The listing builds one solid part. Answer for the finished solid, in the listing's coordinates (mm). Face numbers are marked on the shaded views. A direction names the side the tool comes from. Round coordinates to 2 decimals unless told otherwise and drop trailing zeros. Order: outer loops, then holes, each group sorted by start corner. A loop starts at its lowest first (then second) coordinate and runs counter-clockwise, first axis right, second up. Notation, with made-up numbers: (66.5, -27.75) - (92.5, -27.75) arc R10 cw to (92.5, -15.75) - close; hole circle Ø4 at (75.5, 38). An arc over 180 degrees is marked (long way). One line per item, written item: value. Start each with the question number.
1. A tool of negligible diameter and unlimited length cuts with its end or side. For the marked faces 1, 2 and 3, from which of +Z, -Z, +X, -X, +Y, -Y can it reach the whole face along a straight path? Write none if from no direction.
2. Section C-C, the plane x = 12 is taken. Give the vertices of the cut face in (y, z), then the cut area to 3 significant figures.
3. Section A-A, the plane y = 0 is taken. Give the vertices of the cut face in (x, z), then the cut area to 3 significant figures.
4. Section D-D, the plane z = -6 is taken. Give the vertices of the cut face in (x, y).
5. Straight lines are drawn through the part: line 1 (X direction, y = 0, z = 5.25); line 2 (X direction, y = 0, z = 9.95); line 3 (Y direction, x = 0.5, z = 5.5). For each, find the intervals that lie inside material, in ascending order.
6. Flat-ended cylindrical pins translate along their axes: P1, Ø2, axis at x = 11, y = 11.5, coming from the -Z side; P2, Ø1.5, axis at x = -8.5, z = -16.5, coming from the -Y side; P3, Ø9, axis at x = 3, y = -2, coming from the +Z side. Find the tip coordinate at first contact, or state that the pin passes through.
7. For a pull along X with two mould halves and no side action, classify the marked faces 4, 5 and 6 as released by +X, released by -X, zero draft, split by the parting line, or undercut.
Autodesk Inventor part; units mm, degrees
ref_plane "YZ Plane" through (0, 0, 0) normal (1, 0, 0) x (0, 1, 0)
ref_plane "XZ Plane" through (0, 0, 0) normal (0, 1, 0) x (-1, 0, 0)
ref_plane "XY Plane" through (0, 0, 0) normal (0, 0, 1) x (1, 0, 0)
sketch "Sketch5" plane through (0, 0, 0) normal (1, 0, 0) x (0, 1, 0)
  line L0 (0, 0) -> (17.5, 0)
  line L1 (17.5, 0) -> (17.5, 12.8)
  line L2 (17.5, 12.8) -> (14, 12.8)
  line L3 (14, 12.8) -> (14, 10.3)
  line L4 (14, 10.3) -> (14.7, 10.3)
  line L5 (14.7, 10.3) -> (14.7, 9)
  line L6 (14.7, 9) -> (14, 9)
  line L7 (14, 9) -> (14, 2)
  line L8 (14, 2) -> (8, 2)
  line L9 (8, 2) -> (8, 0)
  line L10 (0, 0) -> (0, 12.8)
  line L11 (9.5, 0) -> (9.5, -25)
  line L12 (9.5, -25) -> (0, -25)
  line L13 (0, -25) -> (0, 0)
  line L14 (8, -25) -> (8, 0)
  dimension "d19" = 17.5
  dimension "d20" = 2.5
  dimension "d21" = 1.3
  dimension "d22" = 7
  dimension "d23" = 2
  dimension "d24" = 14.7
  dimension "d25" = 14
  dimension "d26" = 8
  dimension "d28" = 25
  dimension "d29" = 9.5
  dimension "d30" = 8
revolve "Revolution1" add sketch "Sketch5" angle 360 about axis through (0, 0, 0) along (0, 0, 1) contours L9 L8 L7 L6 L5 L4 L3 L2 L1 L0 | L0 L11 L12 L14
properties part number "P502" material "Aluminum 6061"
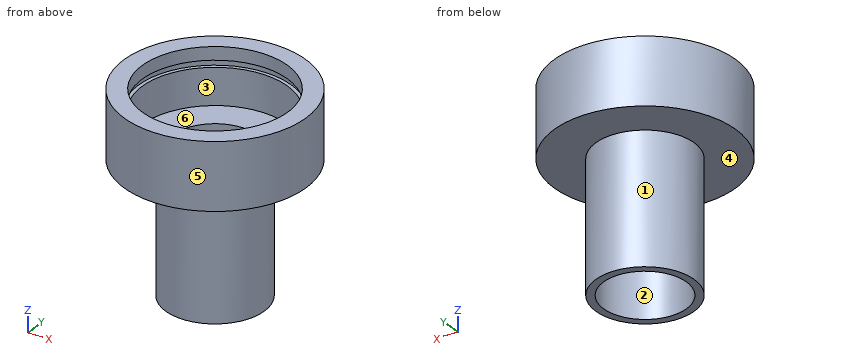
Answer list:
1. face 1: -Z
1. face 2: +Z, -Z
1. face 3: +Z
2. outline: (-12.74, 0) - (12.74, 0) - (12.74, 12.8) - (7.21, 12.8) - (7.21, 10.3) - (8.49, 10.3) - (8.49, 9) - (7.21, 9) - (7.21, 2) - (-7.21, 2) - (-7.21, 9) - (-8.49, 9) - (-8.49, 10.3) - (-7.21, 10.3) - (-7.21, 12.8) - (-12.74, 12.8) - close
2. area: 167 mm²
3. outline: (-17.5, 0) - (-9.5, 0) - (-9.5, -25) - (-8, -25) - (-8, 2) - (-14, 2) - (-14, 9) - (-14.7, 9) - (-14.7, 10.3) - (-14, 10.3) - (-14, 12.8) - (-17.5, 12.8) - close; (8, -25) - (9.5, -25) - (9.5, 0) - (17.5, 0) - (17.5, 12.8) - (14, 12.8) - (14, 10.3) - (14.7, 10.3) - (14.7, 9) - (14, 9) - (14, 2) - (8, 2) - close
3. area: 187 mm²
4. outline: circle Ø19 at (0, 0); hole circle Ø16 at (0, 0)
5. line 1: x = -17.5 to -14, 14 to 17.5
5. line 2: x = -17.5 to -14.7, 14.7 to 17.5
5. line 3: y = -17.49 to -13.99, 13.99 to 17.49
6. P1: stops at z = 0
6. P2: stops at y = -5.49
6. P3: stops at z = 2
7. face 4: zero draft
7. face 5: split by the parting line
7. face 6: undercut
